Read the model definition and answer for the solid it produces. Units are mm, in the model's axes. A direction names the side the tool comes from. Coordinates: 2 decimals unless noted, no trailing zeros. Loops run counter-clockwise (first coordinate to the right, second up) from the corner with the lowest first, then second, coordinate; pieces in that order, holes last. Notation, with made-up numbers: M 47.25,84.5 L 76.25,84.5 A22 ccw 76.25,102.5 Z; hole C -18.75,69.5 d3. An arc over 180 degrees is marked long. Use one line per item in the form item = value. Start each with the question number.
1. Flat-ended cylindrical pins translate along their axes: pin 1 (4 mm diameter, centred on x = -3, y = -5.5, fed in from +Z); pin 2 (3.5 mm diameter, centred on y = 0, z = 10, fed in from -X); pin 3 (1 mm diameter, centred on x = -5.5, z = 10.5, fed in from -Y). Find the tip coordinate at first contact, or state that the pin passes through.
2. The part is cut by section D-D (x = 1.5). Give the vertices of the cut face in (y, z).
3. The part is cut by section A-A (z = 11.25). Give the vertices of the cut face in (x, y).
4. For a pull along X with two mould halves and no side action, classify faces 6 (the flat face through (0.1, -2.899, 4.6)), 7 (the flat face through (0, 1, 5)), 8 (the flat face through (6, 2.2, 10.5)) as released by +X, released by -X, zero draft, split by the parting line, or undercut.
5. The part is cut by section B-B (x = -4.75). Give the vertices of the cut face in (y, z).
6. A tool of negligible diameter and unlimited length cuts with its end or side. For faces 1 (the flat face through (0, 0, 0)), 2 (the cylindrical face through (7.199, -4.66, 2.715)), 3 (the flat face through (3.55, 1, 9)), 4 (the cylindrical face through (-7.215, -4.739, 2.699)), 5 (the flat face through (0, -5, 3)), from which of +Z, -Z, +X, -X, +Y, -Y can it reach the whole face along a straight path? Write none if from no direction.
7. The part is cut by section C-C (y = 2.75). Give the vertices of the cut face in (x, z), plus the area to 3 significant figures.
8. Find the intervals of material crossed by probe 1 along X at (y, z) = (-1, 5.75); probe 2 along Z at (x, y) = (-3.25, -6.5); probe 3 along Y at (x, z) = (-3, 6.5), in increasing order. Write a range as [from, to].
from build123d import *

# Parameters (mm, degrees)
SKETCH_W        = 15
SKETCH_H        = 15
PAD_DEPTH       = 12
SKETCH001_W     = 7.1
SKETCH001_H     = 7.1
POCKET_DEPTH    = 7
POCKET001_DEPTH = 9
CHAMFER_SIZE    = 2
CHAMFER001_SIZE = 3
FILLET_R        = 1


with BuildPart() as part:
    # Sketch → Pad (new body)
    with BuildSketch(Plane.XY):
        Rectangle(SKETCH_W, SKETCH_H)
    extrude(amount=PAD_DEPTH)

    # Sketch001 (on Face6 of Pad) → Pocket (cut)
    with BuildSketch(Plane.XY.offset(12)):
        with Locations((0, 0.650893)):
            Rectangle(SKETCH001_W, SKETCH001_H)
    extrude(amount=-POCKET_DEPTH, mode=Mode.SUBTRACT)

    # Sketch002 (on Face5 of Pocket) → Pocket001 (cut)
    with BuildSketch(Plane.XY.offset(12)):
        Polygon((-3.55, -2.899107), (-7.5, -2.899107), (-7.5, -7.5), (7.5, -7.5), (7.5, -2.899107), (3.55, -2.899107), align=None)
    extrude(amount=-POCKET001_DEPTH, mode=Mode.SUBTRACT)

    # Chamfer
    chamfer_edges = [part.edges().sort_by_distance(p)[0] for p in [
        (0, 7.5, 12),
    ]]
    chamfer(chamfer_edges, length=CHAMFER_SIZE)

    # Chamfer001
    chamfer001_edges = [part.edges().sort_by_distance(p)[0] for p in [
        (-7.5, 1.300446, 12),
        (7.5, 1.300446, 12),
    ]]
    chamfer(chamfer001_edges, length=CHAMFER001_SIZE)

    # Fillet
    fillet_edges = [part.edges().sort_by_distance(p)[0] for p in [
        (7.5, -2.899107, 6),
        (-7.5, -2.899107, 6),
        (-7.5, -5.199554, 3),
        (0, -7.5, 3),
        (7.5, -5.199554, 3),
    ]]
    fillet(fillet_edges, radius=FILLET_R)


solid = part.part
Computed values:
q1.pin_1 = 3
q1.pin_2 = -7.5
q1.pin_3 = -2.9
q2.outline = M -7.5,0 L 7.5,0 L 7.5,10 L 5.5,12 L 4.2,12 L 4.2,5 L -2.9,5 L -2.9,3 L -6.5,3 A1 ccw -7.5,2 Z
q3.outline = M -5.25,-2.9 L -3.55,-2.9 L -3.55,4.2 L 3.55,4.2 L 3.55,-2.9 L 5.25,-2.9 L 5.25,6.25 L -5.25,6.25 Z
q4.face_6 = zero draft
q4.face_7 = undercut
q4.face_8 = released by +X
q5.outline = M -7.5,0 L 7.5,0 L 7.5,10 L 5.75,11.75 L -2.9,11.75 L -2.9,3 L -6.5,3 A1 ccw -7.5,2 Z
q6.face_1 = -Z, +X, -X, +Y, -Y
q6.face_2 = +Z, +X, -Y
q6.face_3 = +Z, -Y
q6.face_4 = +Z, -X, -Y
q6.face_5 = +Z, +X, -X, -Y
q7.outline = M -7.5,0 L 7.5,0 L 7.5,9 L 4.5,12 L 3.55,12 L 3.55,5 L -3.55,5 L -3.55,12 L -4.5,12 L -7.5,9 Z
q7.area = 121 mm²
q8.probe_1 = [-7.5, -3.55], [3.55, 7.5]
q8.probe_2 = [0, 3]
q8.probe_3 = [4.2, 7.5]
